Part model, mm, in its own coordinate system. Face numbers are marked on the shaded views. A direction names the side the tool comes from. Give positions to 0.01 mm unless a question says otherwise; leave off trailing zeros. Order: outer loops, then holes, each group sorted by start corner. A loop starts at its lowest first (then second) coordinate and runs counter-clockwise, first axis right, second up. Notation, with made-up numbers: (64.25, 18.5) -> (79.25, 18.5) arc R16 cw to (79.25, 46.5) -> close; hole circle Ø11 at (57.5, 0). An arc over 180 degrees is marked (long way). Write item = value, one per line. Start each with the question number.
Item 1: Band-saw the part on D-D on z = -3.5. Count the separate pieces of the cut face and the enclosed holes in it, plus the area to 3 significant figures.
Item 2: Band-saw the part on B-B on z = -15. Write the cut outline in (x, y), plus the area to 3 significant figures.
Item 3: Flat gauge pins, fed straight in: P1, Ø3, axis at x = 16.5, z = 2.5, coming from the -Y side; P2, Ø7.5, axis at x = 0, y = -127, coming from the -Z side; P3, Ø4, axis at x = 60, z = 7.5, coming from the -Y side; P4, Ø17, axis at x = 39.31, y = 39.31, coming from the +Z side (3 decimals). Where does each tip first touch, or does it go through?
Item 4: Drill centre lines: line 1 along Y through (x, z) = (34, 4); line 2 along Y through (x, z) = (-127, -1); line 3 along Z through (x, y) = (70, 54) (3 decimals). Where is each one in solid material? Low to high.
Item 5: Band-saw the part on A-A on y = 0. Write the cut outline in (x, z) (3 decimals).
Item 6: Pull direction X, two halves, no side cores. Call the marked faces 3, 4 and 5: +X half, -X half, draft (parallel to the pull), parting line (faces both ways), or undercut.
Item 7: Tool access for the marked faces 1 and 2: list every direction of +Z, -Z, +X, -X, +Y, -Y with a clear straight run to the whole face (end or side of a thin tool).
```python
from build123d import *

# Parameters (mm, degrees)
SKETCH1_R           = 6.35
SKETCH1_R_2         = 14.351
BOSS_EXTRUDE2_DEPTH = 19.05
BOSS_EXTRUDE3_DEPTH = 9.525
FILLET1_R           = 12.7


with BuildPart() as part:
    # Sketch1 → Boss-Extrude2 (new, symmetric)
    with BuildSketch(Plane.XY):
        with BuildLine():
            ThreePointArc((33.959932382, -28.67970524), (30.132939696, -34.801505964), (28.182908549, -41.752742952))
            Line((28.182908549, -41.752742952), (16.670947055, -129.194771817))
            ThreePointArc((16.670947055, -129.194771817), (0, -143.8148), (-16.670947055, -129.194771817))
            Line((-16.670947055, -129.194771817), (-23.40165253, -78.069988022))
            ThreePointArc((-23.40165253, -78.069988022), (-41.457120622, -41.457120622), (-78.069988022, -23.40165253))
            Line((-78.069988022, -23.40165253), (-129.194771817, -16.670947055))
            ThreePointArc((-129.194771817, -16.670947055), (-143.8148, 0), (-129.194771817, 16.670947055))
            Line((-129.194771817, 16.670947055), (-41.752742952, 28.182908549))
            ThreePointArc((-41.752742952, 28.182908549), (-34.801505964, 30.132939696), (-28.67970524, 33.959932382))
            ThreePointArc((-28.67970524, 33.959932382), (31.430896424, 31.430896424), (33.959932382, -28.67970524))
        make_face()
        with Locations(Location((0, -127, 0), (0, 0, 180))):
            Circle(SKETCH1_R, mode=Mode.SUBTRACT)
        with Locations(Location((-127, 0, 0), (0, 0, 180))):
            Circle(SKETCH1_R, mode=Mode.SUBTRACT)
        with Locations(Location((0, 0, 0), (0, 0, 180))):
            Circle(SKETCH1_R_2, mode=Mode.SUBTRACT)
    extrude(amount=BOSS_EXTRUDE2_DEPTH, both=True)

    # Sketch3 → Boss-Extrude3 (add, symmetric)
    with BuildSketch(Plane.XY):
        with BuildLine():
            Line((47.146344636, 83.06736912), (83.06736912, 47.146344636))
            ThreePointArc((83.06736912, 47.146344636), (74.914696381, 12.698674104), (44.182474556, -4.869439613))
            ThreePointArc((44.182474556, -4.869439613), (31.430896424, 31.430896424), (-4.869439613, 44.182474556))
            ThreePointArc((-4.869439613, 44.182474556), (12.698674104, 74.914696381), (47.146344636, 83.06736912))
        make_face()
        with BuildLine():
            Line((25.281244781, 42.070676127), (42.070676127, 25.281244781))
            ThreePointArc((42.070676127, 25.281244781), (49.424803335, 49.424803335), (25.281244781, 42.070676127))
        make_face(mode=Mode.SUBTRACT)
    extrude(amount=BOSS_EXTRUDE3_DEPTH, both=True)

    # Fillet1
    fillet1_edges = [part.edges().sort_by_distance(p)[0] for p in [
        (47.146344636, 83.06736912, 0),
        (-4.869439613, 44.182474556, 0),
        (44.182474556, -4.869439613, 0),
        (83.06736912, 47.146344636, 0),
    ]]
    fillet(fillet1_edges, radius=FILLET1_R)


solid = part.part
```
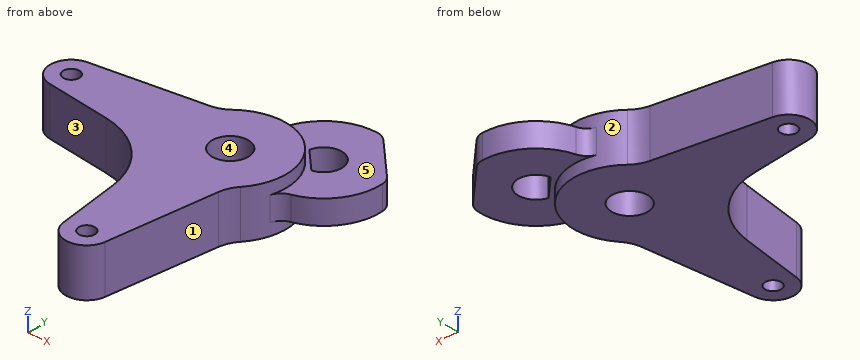
Values found:
q1.separate_pieces = 1
q1.enclosed_holes = 4
q1.area = 18,200 mm^2
q2.outline = (-129.19, -16.67) -> (-78.07, -23.4) arc R63.5 cw to (-23.4, -78.07) -> (-16.67, -129.19) arc R16.81 ccw to (16.67, -129.19) -> (28.18, -41.75) arc R25.4 cw to (33.96, -28.68) arc R44.45 ccw to (-28.68, 33.96) arc R25.4 cw to (-41.75, 28.18) -> (-129.19, 16.67) arc R16.81 ccw to start; hole circle Ø12.7 at (-127, 0); hole circle Ø28.7 at (0, 0); hole circle Ø12.7 at (0, -127)
q2.area = 14,400 mm^2
q3.P1 = -134.6
q3.P2 = through
q3.P3 = -1.02
q3.P4 = 9.525
q4.line_1 = -28.63 to 33.35, 52.59 to 83.44
q4.line_2 = -16.96 to -6.35, 6.35 to 16.96
q4.line_3 = -9.525 to 9.525
q5.outline = (-143.815, -19.05) -> (-133.35, -19.05) -> (-133.35, 19.05) -> (-143.815, 19.05) -> close; (-120.65, -19.05) -> (-14.351, -19.05) -> (-14.351, 19.05) -> (-120.65, 19.05) -> close; (14.351, -19.05) -> (44.45, -19.05) -> (44.45, -9.525) -> (60.056, -9.525) -> (60.056, 9.525) -> (44.45, 9.525) -> (44.45, 19.05) -> (14.351, 19.05) -> close
q6.face_3 = -X half
q6.face_4 = undercut
q6.face_5 = draft
q7.face_1 = +Z, -Z, +X, -Y
q7.face_2 = none
